Source: CAD feature listing. Evaluate the final solid. Frame: model axes, mm. Face numbers are marked on the shaded views. Coordinates: 2 decimals unless noted, no trailing zeros. Order: outer loops, then holes, each group sorted by start corner. A loop starts at its lowest first (then second) coordinate and runs counter-clockwise, first axis right, second up.
Item 1: Section D-D on y = 4. Return the cut outline in (x, z), then the cut area to 3 significant figures.
Item 2: Section B-B on z = -78.5. Return the cut outline in (x, y), then the cut area to 3 significant figures.
Item 3: Mould query, pull axis Z, two halves, no side actions, for the marked faces 1 and 2. Classes: released by +Z, released by -Z, zero draft, split by the parting line, or undercut.
Item 4: Ray query, line 1 (Z direction, x = 156, y = 7); line 2 (Z direction, x = 77, y = -2.05); line 3 (X direction, y = 1, z = -24). Return the intervals inside material, ascending.
Item 5: Contact query for flat-ended pins moving along their axis: P1, Ø2.5, axis at x = 141.8, z = 4, coming from the +Y side; P2, Ø3, axis at y = 4.5, z = -91.5, coming from the +X side; P3, Ø1.5, axis at y = 8, z = -80, coming from the -X side; P4, Ø5, axis at x = 94.5, y = 3.5, coming from the -Z side. Output: stop coordinate, or through.
Item 6: Section C-C on z = -104. Return the cut outline in (x, y).
Item 7: Section A-A on x = 93.2. Return the cut outline in (y, z).
from build123d import *

# Parameters (mm, degrees)
SKETCH1_W           = 166
SKETCH1_H           = 85
SKETCH1_W_2         = 50
SKETCH1_H_2         = 17
BOSS_EXTRUDE4_DEPTH = 10
SKETCH2_W           = 186
SKETCH2_H           = 123
BOSS_EXTRUDE5_DEPTH = 4
SKETCH3_R           = 2
CUT_EXTRUDE2_DEPTH  = 4


with BuildPart() as part:
    # Sketch1 → Boss-Extrude4 (new body)
    with BuildSketch(Plane(origin=(0, 0, 0), x_dir=(1, 0, 0), z_dir=(0, 1, 0))):
        Polygon((0, 89), (116, 89), (116, 108), (170, 108), (170, 89), (170, 0), (0, 0), align=None)
        with Locations((85, 44.5)):
            Rectangle(SKETCH1_W, SKETCH1_H, mode=Mode.SUBTRACT)
        with Locations((143, 97.5)):
            Rectangle(SKETCH1_W_2, SKETCH1_H_2, mode=Mode.SUBTRACT)
    extrude(amount=BOSS_EXTRUDE4_DEPTH)

    # Sketch2 → Boss-Extrude5 (add)
    with BuildSketch(Plane.XZ):
        with Locations((85, -53.5)):
            Rectangle(SKETCH2_W, SKETCH2_H)
    extrude(amount=BOSS_EXTRUDE5_DEPTH)

    # Sketch3 → Cut-Extrude2 (cut)
    with BuildSketch(Plane(origin=(0, 0, 0), x_dir=(1, 0, 0), z_dir=(0, 1, 0))):
        with Locations((-4, -4)):
            Circle(SKETCH3_R)
        with Locations((12.2, -4)):
            Circle(SKETCH3_R)
        with Locations((28.4, -4)):
            Circle(SKETCH3_R)
        with Locations((44.6, -4)):
            Circle(SKETCH3_R)
        with Locations((60.8, -4)):
            Circle(SKETCH3_R)
        with Locations((77, -4)):
            Circle(SKETCH3_R)
        with Locations((93.2, -4)):
            Circle(SKETCH3_R)
        with Locations((109.4, -4)):
            Circle(SKETCH3_R)
        with Locations((125.6, -4)):
            Circle(SKETCH3_R)
        with Locations((141.8, -4)):
            Circle(SKETCH3_R)
        with Locations((158, -4)):
            Circle(SKETCH3_R)
        with Locations((174.2, -4)):
            Circle(SKETCH3_R)
        with Locations((174.2, 12.5)):
            Circle(SKETCH3_R)
        with Locations((174.2, 29)):
            Circle(SKETCH3_R)
        with Locations((174.2, 45.5)):
            Circle(SKETCH3_R)
        with Locations((174.2, 62)):
            Circle(SKETCH3_R)
        with Locations((174.2, 78.5)):
            Circle(SKETCH3_R)
        with Locations((174.2, 95)):
            Circle(SKETCH3_R)
        with Locations((12.2, 111.5)):
            Circle(SKETCH3_R)
        with Locations((28.4, 111.5)):
            Circle(SKETCH3_R)
        with Locations((44.6, 111.5)):
            Circle(SKETCH3_R)
        with Locations((60.8, 111.5)):
            Circle(SKETCH3_R)
        with Locations((77, 111.5)):
            Circle(SKETCH3_R)
        with Locations((93.2, 111.5)):
            Circle(SKETCH3_R)
        with Locations((109.4, 111.5)):
            Circle(SKETCH3_R)
        with Locations((125.6, 111.5)):
            Circle(SKETCH3_R)
        with Locations((141.8, 111.5)):
            Circle(SKETCH3_R)
        with Locations((158, 111.5)):
            Circle(SKETCH3_R)
        with Locations((174.2, 111.5)):
            Circle(SKETCH3_R)
        with Locations((-4, 12.5)):
            Circle(SKETCH3_R)
        with Locations((-4, 29)):
            Circle(SKETCH3_R)
        with Locations((-4, 45.5)):
            Circle(SKETCH3_R)
        with Locations((-4, 62)):
            Circle(SKETCH3_R)
        with Locations((-4, 78.5)):
            Circle(SKETCH3_R)
        with Locations((-4, 95)):
            Circle(SKETCH3_R)
        with Locations((-4, 111.5)):
            Circle(SKETCH3_R)
    extrude(amount=-CUT_EXTRUDE2_DEPTH, mode=Mode.SUBTRACT)


solid = part.part
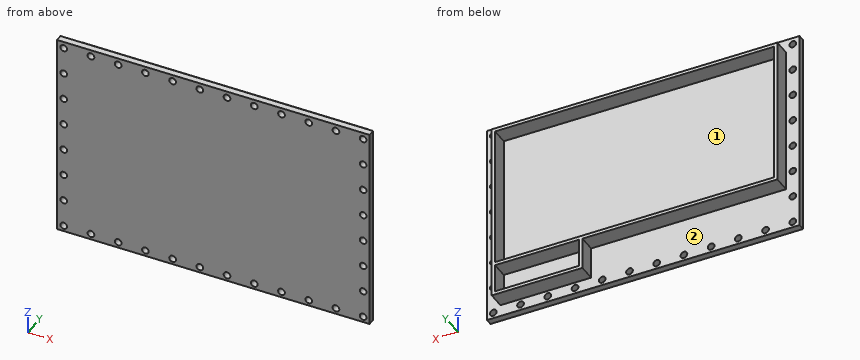
Answer list:
1. outline: (0, -89) - (116, -89) - (116, -108) - (170, -108) - (170, 0) - (0, 0) - close; hole (2, -87) - (168, -87) - (168, -2) - (2, -2) - close; hole (118, -106) - (168, -106) - (168, -89) - (118, -89) - close
1. area: 1,200 mm2
2. outline: (-8, -4) - (-6, -4) - (-6, 0) - (-8, 0) - close; (-2, -4) - (172.2, -4) - (172.2, 0) - (170, 0) - (170, 10) - (168, 10) - (168, 0) - (2, 0) - (2, 10) - (0, 10) - (0, 0) - (-2, 0) - close; (176.2, -4) - (178, -4) - (178, 0) - (176.2, 0) - close
2. area: 752 mm2
3. face 1: undercut
3. face 2: zero draft
4. line 1: z = -108 to -106, -89 to -87, -2 to 0
4. line 2: z = -115 to -113.5, -109.5 to 2, 6 to 8
4. line 3: x = 0 to 2, 168 to 170
5. P1: passes through
5. P2: stops at x = 170
5. P3: stops at x = 0
5. P4: stops at z = -89
6. outline: (-8, -4) - (178, -4) - (178, 0) - (170, 0) - (170, 10) - (168, 10) - (168, 0) - (118, 0) - (118, 10) - (116, 10) - (116, 0) - (-8, 0) - close
7. outline: (-4, -115) - (0, -115) - (0, -113.5) - (-4, -113.5) - close; (-4, -109.5) - (0, -109.5) - (0, -89) - (10, -89) - (10, -87) - (0, -87) - (0, -2) - (10, -2) - (10, 0) - (0, 0) - (0, 2) - (-4, 2) - close; (-4, 6) - (0, 6) - (0, 8) - (-4, 8) - close
